from build123d import *

# Parameters (mm, degrees)
CROQUIS1_R              = 9.525
SALIENTE_EXTRUIR1_DEPTH = 20
CROQUIS2_R              = 31.75
SALIENTE_EXTRUIR2_DEPTH = 380
CROQUIS3_R              = 9.525
SALIENTE_EXTRUIR3_DEPTH = 20
SALIENTE_EXTRUIR4_DEPTH = 20


with BuildPart() as part:
    # Croquis1 → Saliente-Extruir1 (new body)
    with BuildSketch(Plane(origin=(0, 0, 0), x_dir=(0, 0, -1), z_dir=(1, 0, 0))):
        Circle(CROQUIS1_R)
    extrude(amount=SALIENTE_EXTRUIR1_DEPTH)

    # Croquis2 → Saliente-Extruir2 (add)
    with BuildSketch(Plane(origin=(20, 0, 0), x_dir=(0, 0, -1), z_dir=(1, 0, 0))):
        Circle(CROQUIS2_R)
    extrude(amount=SALIENTE_EXTRUIR2_DEPTH)

    # Croquis3 → Saliente-Extruir3 (add)
    with BuildSketch(Plane(origin=(400, 0, 0), x_dir=(0, 0, -1), z_dir=(1, 0, 0))):
        Circle(CROQUIS3_R)
    extrude(amount=SALIENTE_EXTRUIR3_DEPTH)

    # Croquis4 → Saliente-Extruir4 (add)
    with BuildSketch(Plane.ZY):
        Polygon((0, 9.525), (-1, 9.525), (-1, 8.525), (1, 8.525), (1, 9.525), align=None)
        Polygon((9.525, 0), (9.525, 1), (8.525, 1), (8.525, -1), (9.525, -1), align=None)
    extrude(amount=-SALIENTE_EXTRUIR4_DEPTH)


solid = part.part
For this review, take the finished solid that the model builds, in its own axes (mm). A direction names the side the tool comes from. Round coordinates to 2 decimals unless told otherwise and drop trailing zeros. Order: outer loops, then holes, each group sorted by start corner. A loop starts at its lowest first (then second) coordinate and runs counter-clockwise, first axis right, second up. Notation, with made-up numbers: (4, -5) -> (38, -5) arc R22 cw to (38, 30) -> close; hole circle Ø7 at (65, -29.5). An arc over 180 degrees is marked (long way). Put each result on its own line as item: value.
Q1. Machinability: for faces 1 (the cylindrical face through (9.86, 6.8, 6.67)), 2 (the flat face through (420, 0, 0)), 3 (the flat face through (0, 0, 0)), 4 (the flat face through (20, 8, -7)), 5 (the flat face through (400, 8, -7)), which of the approach directions +Z, -Z, +X, -X, +Y, -Y give a long, thin tool a straight path to every point of the face, cutting with its end or side? Answer none if there is none.
Check result:
face 1: +Z, -X, +Y
face 2: +Z, -Z, +X, +Y, -Y
face 3: +Z, -Z, -X, +Y, -Y
face 4: -X
face 5: +X
Q2. Add section A-A on x = 110. Write out the cut boundary in (y, z).
Check result:
outline: circle Ø63.5 at (0, 0)
Q3. Add section B-B on z = -22.5. Write out the cut boundary in (x, y).
Check result:
outline: (20, -22.4) -> (400, -22.4) -> (400, 22.4) -> (20, 22.4) -> close
Q4. For probe 1 along Y at (x, z) = (80.5, 0); probe 2 along X at (y, z) = (-27.5, -2); probe 3 along Z at (x, y) = (345, 27), list the stretches that pass through material, from the lowest coordinate up. Write a range as [from, to].
Check result:
probe 1: [-31.75, 31.75]
probe 2: [20, 400]
probe 3: [-16.71, 16.71]
Q5. Insertion check: pin 1 Ø3 at (x, z) = (43.5, 21) entering from -Y; pin 2 Ø5 at (y, z) = (-3, 12.5) entering from -X; pin 3 Ø3 at (x, y) = (271.5, -21) entering from -Z. Each pin has a flat end and moves straight along its axis. Give the tip position at first contact, or say it passes through.
Check result:
pin 1: y = -25.06
pin 2: x = 20
pin 3: z = -25.06
Q6. Add section C-C on y = 20.5. Write out the cut boundary in (x, z), plus the area to 3 significant figures.
Check result:
outline: (20, -24.24) -> (400, -24.24) -> (400, 24.24) -> (20, 24.24) -> close
area: 18,400 mm2
